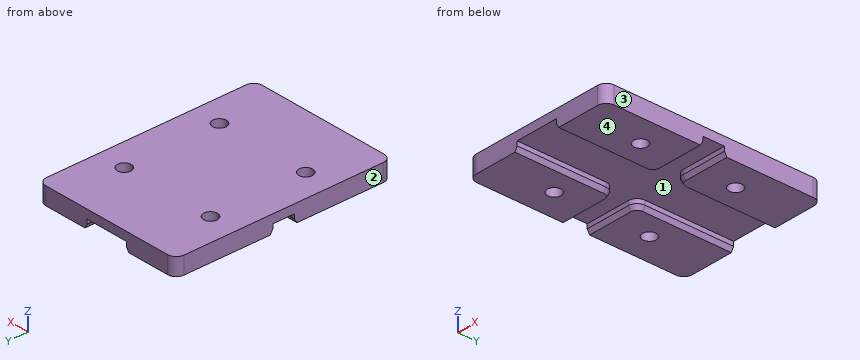
from build123d import *
from OCP.BRepFilletAPI import BRepFilletAPI_MakeChamfer

# Parameters (mm, degrees)
SCHIZZO1_W                   = 35
SCHIZZO1_H                   = 50
ESTRUSIONE_ESTRUSIONE1_DEPTH = 2
TAGLIO_ESTRUSIONE1_DEPTH     = 2
RACCORDO1_R                  = 2
SMUSSO1_SIZE                 = 1
SMUSSO1_SIZE2                = 0.577350269
SKETCH1_R                    = 1.6
CUT_EXTRUDE1_DEPTH           = 31.777426793
CUT_EXTRUDE1_DEPTH_BACK      = 31.777426793


with BuildPart() as part:
    # Schizzo1 → Estrusione-Estrusione1 (new, symmetric)
    with BuildSketch(Plane.XY):
        Rectangle(SCHIZZO1_W, SCHIZZO1_H)
    extrude(amount=ESTRUSIONE_ESTRUSIONE1_DEPTH, both=True)

    # Schizzo2 → Taglio-Estrusione1 (cut)
    with BuildSketch(Plane(origin=(0, 0, -2), x_dir=(-1, 0, 0), z_dir=(0, 0, -1))):
        Polygon((-5, -25), (5, -25), (5, -2.5), (17.5, -2.5), (17.5, 2.5), (5, 2.5), (5, 25), (-5, 25), (-5, 2.5), (-17.5, 2.5), (-17.5, -2.5), (-5, -2.5), align=None)
    extrude(amount=-TAGLIO_ESTRUSIONE1_DEPTH, mode=Mode.SUBTRACT)

    # Raccordo1
    raccordo1_edges = [part.edges().sort_by_distance(p)[0] for p in [
        (-5, 2.5, -1),
        (-5, -2.5, -1),
        (5, -2.5, -1),
        (5, 2.5, -1),
        (-17.5, -25, 0),
        (17.5, -25, 0),
        (17.5, 25, 0),
        (-17.5, 25, 0),
    ]]
    fillet(raccordo1_edges, radius=RACCORDO1_R)

    # Smusso1: one chamfer whose edges measure the first distance from different faces: ONE call of the kernel's chamfer builder (chamfer() names one face for all edges)
    smusso1_edges_1 = [part.edges().sort_by_distance(p)[0] for p in [
        (5, 14.75, -2),
    ]]
    smusso1_side_1 = [part.faces().sort_by_distance(p)[0] for p in [
        (5, 14.75, -1),
    ]]
    smusso1_edges_2 = [part.edges().sort_by_distance(p)[0] for p in [
        (12.25, -2.5, -2),
    ]]
    smusso1_side_2 = [part.faces().sort_by_distance(p)[0] for p in [
        (12.25, -2.5, -1),
    ]]
    smusso1_edges_3 = [part.edges().sort_by_distance(p)[0] for p in [
        (-5, -14.75, -2),
    ]]
    smusso1_side_3 = [part.faces().sort_by_distance(p)[0] for p in [
        (-5, -14.75, -1),
    ]]
    smusso1_edges_4 = [part.edges().sort_by_distance(p)[0] for p in [
        (-12.25, 2.5, -2),
    ]]
    smusso1_side_4 = [part.faces().sort_by_distance(p)[0] for p in [
        (-12.25, 2.5, -1),
    ]]
    smusso1_edges_5 = [part.edges().sort_by_distance(p)[0] for p in [
        (5, -14.75, -2),
    ]]
    smusso1_side_5 = [part.faces().sort_by_distance(p)[0] for p in [
        (5, -14.75, -1),
    ]]
    smusso1_edges_6 = [part.edges().sort_by_distance(p)[0] for p in [
        (5.585786438, -3.085786438, -2),
    ]]
    smusso1_side_6 = [part.faces().sort_by_distance(p)[0] for p in [
        (5.585786438, -3.085786438, -1),
    ]]
    smusso1_edges_7 = [part.edges().sort_by_distance(p)[0] for p in [
        (-5, 14.75, -2),
    ]]
    smusso1_side_7 = [part.faces().sort_by_distance(p)[0] for p in [
        (-5, 14.75, -1),
    ]]
    smusso1_edges_8 = [part.edges().sort_by_distance(p)[0] for p in [
        (-5.585786438, 3.085786438, -2),
    ]]
    smusso1_side_8 = [part.faces().sort_by_distance(p)[0] for p in [
        (-5.585786438, 3.085786438, -1),
    ]]
    smusso1_edges_9 = [part.edges().sort_by_distance(p)[0] for p in [
        (-12.25, -2.5, -2),
    ]]
    smusso1_side_9 = [part.faces().sort_by_distance(p)[0] for p in [
        (-12.25, -2.5, -1),
    ]]
    smusso1_edges_10 = [part.edges().sort_by_distance(p)[0] for p in [
        (-5.585786438, -3.085786438, -2),
    ]]
    smusso1_side_10 = [part.faces().sort_by_distance(p)[0] for p in [
        (-5.585786438, -3.085786438, -1),
    ]]
    smusso1_edges_11 = [part.edges().sort_by_distance(p)[0] for p in [
        (12.25, 2.5, -2),
    ]]
    smusso1_side_11 = [part.faces().sort_by_distance(p)[0] for p in [
        (12.25, 2.5, -1),
    ]]
    smusso1_edges_12 = [part.edges().sort_by_distance(p)[0] for p in [
        (5.585786438, 3.085786438, -2),
    ]]
    smusso1_side_12 = [part.faces().sort_by_distance(p)[0] for p in [
        (5.585786438, 3.085786438, -1),
    ]]
    smusso1 = BRepFilletAPI_MakeChamfer(part.part.solid().wrapped)
    for e in smusso1_edges_1:
        smusso1.Add(SMUSSO1_SIZE, SMUSSO1_SIZE2, e.wrapped, smusso1_side_1[0].wrapped)  # the first distance lies on this face
    for e in smusso1_edges_2:
        smusso1.Add(SMUSSO1_SIZE, SMUSSO1_SIZE2, e.wrapped, smusso1_side_2[0].wrapped)  # the first distance lies on this face
    for e in smusso1_edges_3:
        smusso1.Add(SMUSSO1_SIZE, SMUSSO1_SIZE2, e.wrapped, smusso1_side_3[0].wrapped)  # the first distance lies on this face
    for e in smusso1_edges_4:
        smusso1.Add(SMUSSO1_SIZE, SMUSSO1_SIZE2, e.wrapped, smusso1_side_4[0].wrapped)  # the first distance lies on this face
    for e in smusso1_edges_5:
        smusso1.Add(SMUSSO1_SIZE, SMUSSO1_SIZE2, e.wrapped, smusso1_side_5[0].wrapped)  # the first distance lies on this face
    for e in smusso1_edges_6:
        smusso1.Add(SMUSSO1_SIZE, SMUSSO1_SIZE2, e.wrapped, smusso1_side_6[0].wrapped)  # the first distance lies on this face
    for e in smusso1_edges_7:
        smusso1.Add(SMUSSO1_SIZE, SMUSSO1_SIZE2, e.wrapped, smusso1_side_7[0].wrapped)  # the first distance lies on this face
    for e in smusso1_edges_8:
        smusso1.Add(SMUSSO1_SIZE, SMUSSO1_SIZE2, e.wrapped, smusso1_side_8[0].wrapped)  # the first distance lies on this face
    for e in smusso1_edges_9:
        smusso1.Add(SMUSSO1_SIZE, SMUSSO1_SIZE2, e.wrapped, smusso1_side_9[0].wrapped)  # the first distance lies on this face
    for e in smusso1_edges_10:
        smusso1.Add(SMUSSO1_SIZE, SMUSSO1_SIZE2, e.wrapped, smusso1_side_10[0].wrapped)  # the first distance lies on this face
    for e in smusso1_edges_11:
        smusso1.Add(SMUSSO1_SIZE, SMUSSO1_SIZE2, e.wrapped, smusso1_side_11[0].wrapped)  # the first distance lies on this face
    for e in smusso1_edges_12:
        smusso1.Add(SMUSSO1_SIZE, SMUSSO1_SIZE2, e.wrapped, smusso1_side_12[0].wrapped)  # the first distance lies on this face
    add(Compound.cast(smusso1.Shape()), mode=Mode.REPLACE)

    # Sketch1 → Cut-Extrude1 (cut, two sides)
    with BuildSketch(Plane.XY.offset(2)) as cut_extrude1_sk:
        with Locations((-11, 11)):
            Circle(SKETCH1_R)
        with Locations(Location((11, 11, 0), (0, 0, 180))):
            Circle(SKETCH1_R)
        with Locations((11, -11)):
            Circle(SKETCH1_R)
        with Locations(Location((-11, -11, 0), (0, 0, 180))):
            Circle(SKETCH1_R)
    extrude(amount=CUT_EXTRUDE1_DEPTH, mode=Mode.SUBTRACT)
    extrude(cut_extrude1_sk.sketch, amount=-CUT_EXTRUDE1_DEPTH_BACK, mode=Mode.SUBTRACT)


solid = part.part
The listing builds one solid part. Answer for the finished solid, in the listing's coordinates (mm). Face numbers are marked on the shaded views. Coordinates: 2 decimals unless noted, no trailing zeros. Write each loop counter-clockwise with the first axis right and the second up, starting at its lowest first coordinate (ties: lowest second). Pieces come first, ordered by that corner, then holes. Notation, with made-up numbers: M -12,-31 L 17,-31 A27 cw 17,-15 Z; hole C 52,73 d11. An arc over 180 degrees is marked long. Use one line per item in the form item = value.
Item 1: Find section A-A, the plane x = -11. Give the vertices of the cut face in (y, z).
Model answer:
outline = M -25,-2 L -12.6,-2 L -12.6,2 L -25,2 Z; M -9.4,-2 L -3.08,-2 L -2.5,-1 L -2.5,0 L 2.5,0 L 2.5,-1 L 3.08,-2 L 9.4,-2 L 9.4,2 L -9.4,2 Z; M 12.6,-2 L 25,-2 L 25,2 L 12.6,2 Z
Item 2: Find the intervals of material crossed by probe 1 along Y at (x, z) = (-11, -1); probe 2 along Y at (x, z) = (11, 1.1); probe 3 along X at (y, z) = (14.5, -0.4), in increasing order.
Model answer:
probe_1 = -25 to -12.6, -9.4 to -2.5, 2.5 to 9.4, 12.6 to 25
probe_2 = -25 to -12.6, -9.4 to 9.4, 12.6 to 25
probe_3 = -17.5 to -5, 5 to 17.5
Item 3: Find section C-C, the plane z = 0.6. Give the vertices of the cut face in (x, y), plus the area to 3 significant figures.
Model answer:
outline = M -17.5,-23 A2 ccw -15.5,-25 L 15.5,-25 A2 ccw 17.5,-23 L 17.5,23 A2 ccw 15.5,25 L -15.5,25 A2 ccw -17.5,23 Z; hole C -11,-11 d3.2; hole C -11,11 d3.2; hole C 11,-11 d3.2; hole C 11,11 d3.2
area = 1,710 mm2
Item 4: The mould has two halves that part along X. Classify the marked faces 1, 2, 3 and 4: released by +X, released by -X, zero draft, split by the parting line, or undercut.
Model answer:
face_1 = undercut
face_2 = released by -X
face_3 = released by +X
face_4 = zero draft
Item 5: Find section D-D, the plane y = 15. Give the vertices of the cut face in (x, z).
Model answer:
outline = M -17.5,-2 L -5.58,-2 L -5,-1 L -5,0 L 5,0 L 5,-1 L 5.58,-2 L 17.5,-2 L 17.5,2 L -17.5,2 Z
Item 6: Given P1, Ø10.5, axis at x = -3.5, y = 0.5, coming from the -Z side, flat-ended and moving along its own axis, determine where the tip first touches the part or whether it passes through.
Model answer:
P1 = -2
Item 7: Find section B-B, the plane y = -11. Give the vertices of the cut face in (x, z).
Model answer:
outline = M -17.5,-2 L -12.6,-2 L -12.6,2 L -17.5,2 Z; M -9.4,-2 L -5.58,-2 L -5,-1 L -5,0 L 5,0 L 5,-1 L 5.58,-2 L 9.4,-2 L 9.4,2 L -9.4,2 Z; M 12.6,-2 L 17.5,-2 L 17.5,2 L 12.6,2 Z
